Here's how the part is built. I have some questions about the finished solid (model axes, mm). Face numbers are marked on the shaded views. A direction names the side the tool comes from. Coordinates: 2 decimals unless noted, no trailing zeros. Write each loop counter-clockwise with the first axis right and the second up, starting at its lowest first coordinate (ties: lowest second). Pieces come first, ordered by that corner, then holes.
(1) Imagine slicing it at B-B, the plane x = 0. List the corners of the cut face in (y, z) for me.
(2) For pin 1 Ø1.5 at (y, z) = (-2, -1.5) entering from +X; pin 2 Ø3.5 at (x, y) = (0, 0.5) entering from +Z, each with a flat end and sliding along its axis, tell me the tip position at first contact or that it passes through.
(3) Which directions (+Z, -Z, +X, -X, +Y, -Y) give clear straight access to the entire face, cutting with the end or side of a thin tool? Please do the marked faces 4 and 5.
(4) Imagine slicing it at A-A, the plane z = -2.25. List the corners of the cut face in (x, y) for me, plus the area to 3 significant figures.
(5) Please list where these lines run through material, in increasing order: probe 1 along X at (y, z) = (-1.5, -3.5); probe 2 along Y at (x, z) = (-0.75, -5.5); probe 3 along X at (y, z) = (1.75, -2).
(6) Thinking about a two-plate mould opening in Y: for the marked faces 1, 2 and 3, which applies, released by +Y, released by -Y, zero draft, split by the parting line, or undercut?
```python
from build123d import *

# Parameters (mm, degrees)
BOSS_EXTRUDE1_DEPTH = 4.4


with BuildPart() as part:
    # Sketch1 → Boss-Extrude1 (new body)
    with BuildSketch(Plane.XY):
        Polygon((4.618802154, 0), (2.309401077, 4), (-2.309401077, 4), (-4.618802154, 0), (-2.309401077, -4), (2.309401077, -4), align=None)
    extrude(amount=-BOSS_EXTRUDE1_DEPTH)

    # Sketch2 → Revolve1 (revolve)
    with BuildSketch(Plane(origin=(0, 0, 0), x_dir=(0, 0, -1), z_dir=(1, 0, 0))):
        with BuildLine():
            Line((4.4, 2), (6.011274944, 2))
            Line((6.011274944, 2), (6.011274944, 2.25))
            Line((6.011274944, 2.25), (6.161274944, 2.25))
            ThreePointArc((6.161274944, 2.25), (6.259368372, 2.290631628), (6.3, 2.388725056))
            ThreePointArc((6.3, 2.388725056), (6.04773841, 2.99773841), (5.438725056, 3.25))
            Line((5.438725056, 3.25), (4.841008238, 3.302293446))
            ThreePointArc((4.841008238, 3.302293446), (4.608464966, 3.340201362), (4.4, 3.45))
            Line((4.4, 3.45), (4.4, 2))
        make_face()
    revolve(axis=Axis((0, 0, 11.954173971), (0, 0, -1)))

    # Sketch3 → Cut-Revolve1 (revolve, cut)
    with BuildSketch(Plane(origin=(0, 0, 0), x_dir=(1, 0, 0), z_dir=(0, 1, 0))):
        Polygon((-3.45, 4.4), (-4.618802154, 3.725191762), (-4.618802154, 4.4), align=None)
        Polygon((-3.45, 0), (-4.618802154, 0.674808238), (-4.618802154, 0), align=None)
    revolve(axis=Axis((0, 0, 0), (0, 0, -1)), mode=Mode.SUBTRACT)

    # Sketch4 → Cut-Revolve2 (revolve, cut)
    with BuildSketch(Plane(origin=(0, 0, 0), x_dir=(0, 0, -1), z_dir=(1, 0, 0))):
        Polygon((0, 2.55), (0.45, 2.1), (4.4, 2.1), (4.4, 0), (0, 0), align=None)
    revolve(axis=Axis((0, 0, 1.412389309), (0, 0, -1)), mode=Mode.SUBTRACT)


solid = part.part
```
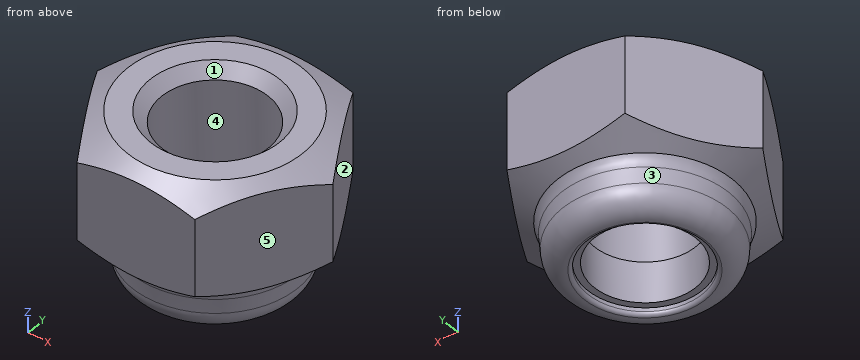
Recorded:
1. outline: (-4, -4.08) - (-3.45, -4.4) arc R0.73 cw to (-3.3, -4.84) - (-3.25, -5.44) arc R0.86 ccw to (-2.39, -6.3) arc R0.14 ccw to (-2.25, -6.16) - (-2.25, -6.01) - (-2, -6.01) - (-2, -4.4) - (-2.1, -4.4) - (-2.1, -0.45) - (-2.55, 0) - (-3.45, 0) - (-4, -0.32) - close; (2, -6.01) - (2.25, -6.01) - (2.25, -6.16) arc R0.14 ccw to (2.39, -6.3) arc R0.86 ccw to (3.25, -5.44) - (3.3, -4.84) arc R0.73 cw to (3.45, -4.4) - (4, -4.08) - (4, -0.32) - (3.45, 0) - (2.55, 0) - (2.1, -0.45) - (2.1, -4.4) - (2, -4.4) - close
2. pin 1: stops at x = 3.9
2. pin 2: stops at z = -0.3
3. face 4: +Z
3. face 5: +Z, -Z, +X, -Y
4. outline: (-4.62, 0) - (-2.31, -4) - (2.31, -4) - (4.62, 0) - (2.31, 4) - (-2.31, 4) - close; hole circle Ø4.2 at (0, 0)
4. area: 41.6 mm2
5. probe 1: x = -3.75 to -1.47, 1.47 to 3.75
5. probe 2: y = -3.16 to -1.85, 1.85 to 3.16
5. probe 3: x = -3.61 to -1.16, 1.16 to 3.61
6. face 1: undercut
6. face 2: released by +Y
6. face 3: split by the parting line
